Check sheet for the drawn part. Datum: minimum x, y, z corner. Units: mm. A direction names the side the tool comes from. Give positions to 0.01 mm unless a question says otherwise; leave off trailing zeros. Loops run counter-clockwise (first coordinate to the right, second up) from the corner with the lowest first, then second, coordinate; pieces in that order, holes last. Notation, with made-up numbers: (79.5, 25) - (83.5, 25) arc R30 ccw to (83.5, 55) - close; hole circle Ø6 at (47, 27.25). An arc over 180 degrees is marked (long way). Answer in a Markdown table with one row per item.
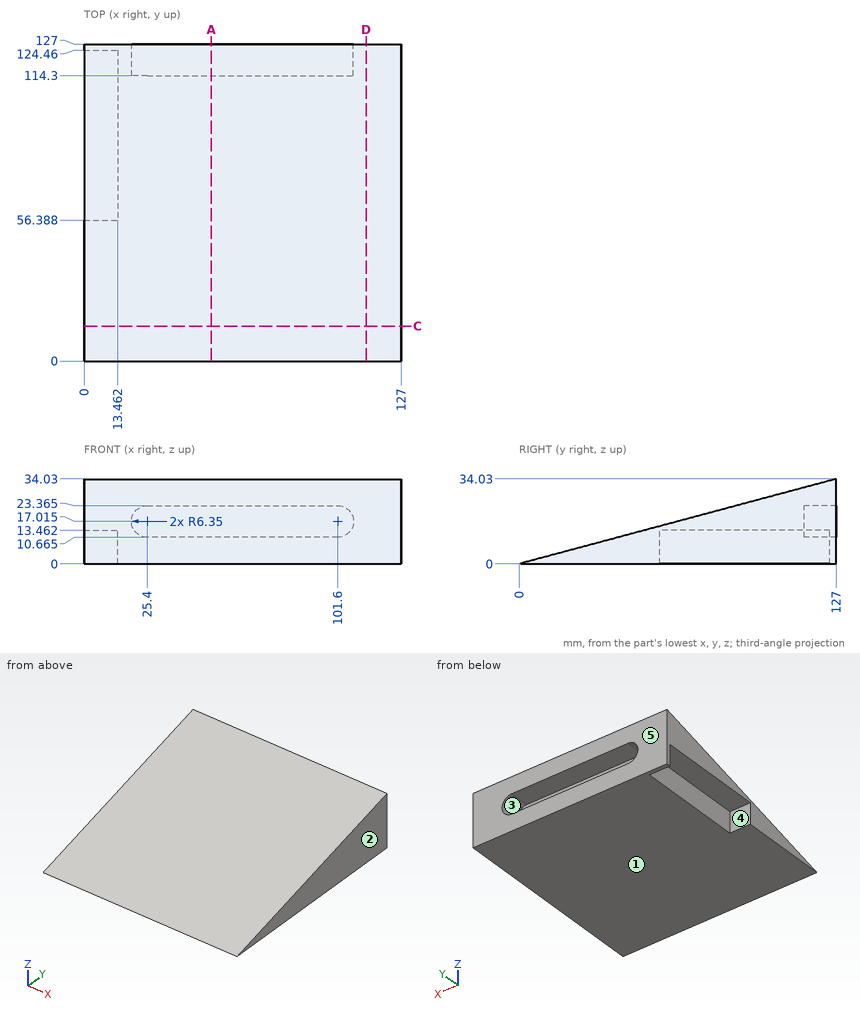
Q1. Thickness scan on line 1 (X direction, y = 59.5, z = 11); line 2 (X direction, y = 122, z = 16); line 3 (Z direction, x = 78, y = 81) (1 decimal). Record the ranges inside material, lowest first.
Completed:
| item | result |
|---|---|
| line 1 | 13.46 to 127 |
| line 2 | 0 to 19.13, 107.87 to 127 |
| line 3 | 0 to 21.7 |
Q2. Sectioned sample at D-D (x = 113). Record the cut outline in (y, z).
Completed:
| item | result |
|---|---|
| outline | (0, 0) - (127, 0) - (127, 34.03) - close |
Q3. Sectioned sample at A-A (x = 51). Record the cut outline in (y, z) (1 decimal), and give its area (3 significant figures).
Completed:
| item | result |
|---|---|
| outline | (0, 0) - (127, 0) - (127, 10.7) - (114.3, 10.7) - (114.3, 23.4) - (127, 23.4) - (127, 34) - close |
| area | 2,000 mm^2 |
Q4. Draft check along X on the marked faces 1, 2 and 3. Enter one of: +X half, -X half, draft (parallel to the pull), parting line (faces both ways), or undercut.
Completed:
| item | result |
|---|---|
| face 1 | draft |
| face 2 | +X half |
| face 3 | undercut |
Q5. Tool access check on the marked faces 4 and 5. Record the directions out of +Z, -Z, +X, -X, +Y, -Y that give a thin tool (end or side, any length) a straight path to the whole face; none if there is none.
Completed:
| item | result |
|---|---|
| face 4 | -Z, -X |
| face 5 | +Z, -Z, +X, -X, +Y |
Q6. Sectioned sample at C-C (y = 14). Record the cut outline in (x, z).
Completed:
| item | result |
|---|---|
| outline | (0, 0) - (127, 0) - (127, 3.75) - (0, 3.75) - close |
Q7. Go/stop test with flat-tipped pins: P1, Ø4, axis at x = 80, z = 17.5, coming from the +Y side; P2, Ø3, axis at x = 107.5, y = 25.5, coming from the +Z side (1 decimal); P3, Ø4, axis at x = 3.5, y = 80, coming from the -Z side. Record where each tip stops, or that it passes through.
Completed:
| item | result |
|---|---|
| P1 | y = 114.3 |
| P2 | z = 7.2 |
| P3 | z = 13.46 |
